Could you check a few things on this model? Use its own coordinates, in mm. Coordinates: 2 decimals unless noted, no trailing zeros. Use a Markdown table: item, result. Add a question column.
1) If I drill on L1, parallel to Z at x = -36.5, y = 3; L2, parallel to Y at x = -26, z = 5.5; L3, parallel to X at y = 2.75, z = 7.5, over which ranges is the centre line in solid material (lowest first)? Write a range as [from, to].
2) Thinking about a two-plate mould opening in Z: for faces 1 (the flat face through (-1, 5, 70)), 2 (the cylindrical face through (-8.67, 2.46, -39.05)), 3 (the flat face through (1, 5, -70)), 4 (the flat face through (-1, 5, 1)), which applies, +Z half, -Z half, draft (parallel to the pull), parting line (faces both ways), or undercut?
3) Will these pins go through, and if not, where does the flat tip stop? pin 1 Ø3 at (x, y) = (29.5, 7.5) entering from +Z; pin 2 Ø4 at (y, z) = (4.5, -26.5) entering from -X; pin 3 Ø24 at (x, z) = (12, 15.5) entering from -Y.
Autodesk Inventor part; units mm, degrees
ref_plane "YZ Plane" through (0, 0, 0) normal (1, 0, 0) x (0, 1, 0)
ref_plane "XZ Plane" through (0, 0, 0) normal (0, 1, 0) x (-1, 0, 0)
ref_plane "XY Plane" through (0, 0, 0) normal (0, 0, 1) x (1, 0, 0)
sketch "Sketch1" plane through (0, 0, 0) normal (0, 1, 0) x (-1, 0, 0)
  line L0 (75, -75) -> (-75, -75)
  line L1 (-75, -75) -> (-75, 75)
  line L2 (-75, 75) -> (75, 75)
  line L3 (75, 75) -> (75, -75)
  line L4 (75, -75) -> (-75, 75) construction
  line L5 (-75, -75) -> (75, 75) construction
  point P0 (0, 0)
  dimension "d0" = 150
  dimension "d1" = 150
extrude "Extrusion1" add sketch "Sketch1" along normal blind 10
chamfer "Chamfer1" distance 10 angle 45 4 edges at (0, 10, 75) (-75, 10, 0) (0, 10, -75) (75, 10, 0)
sketch "Sketch2" plane through (0, 0, 0) normal (0, -1, 0) x (1, 0, 0)
  circle A0 centre (0, 0) radius 40
  dimension "d7" = 80
extrude "Extrusion2" cut sketch "Sketch2" against normal blind 5
properties part number "side"
Answer sheet:
| question | item | result |
|---|---|---|
| 1 | L1 | [-72, -16.36], [16.36, 72] |
| 1 | L2 | [5, 10] |
| 1 | L3 | [-72.25, -39.29], [39.29, 72.25] |
| 2 | face 1 | +Z half |
| 2 | face 2 | undercut |
| 2 | face 3 | -Z half |
| 2 | face 4 | undercut |
| 3 | pin 1 | z = 69 |
| 3 | pin 2 | x = -72.5 |
| 3 | pin 3 | y = 5 |
